from build123d import *

# Parameters (mm, degrees)
F0_W     = 40
F0_H     = 40
F1_DEPTH = 1550
F2_R     = 6.5
F3_DEPTH = 10
F4_R     = 6.5
F5_DEPTH = 10


with BuildPart() as f1:
    # F0 (on Top) → F1 (new body)
    with BuildSketch(Plane.XY):
        with BuildLine():
            Line((-20, -25), (20, -25))
            ThreePointArc((20, -25), (23.535534, -23.535534), (25, -20))
            Line((25, -20), (25, 20))
            ThreePointArc((25, 20), (23.535534, 23.535534), (20, 25))
            Line((20, 25), (-20, 25))
            ThreePointArc((-20, 25), (-23.535534, 23.535534), (-25, 20))
            Line((-25, 20), (-25, -20))
            ThreePointArc((-25, -20), (-23.535534, -23.535534), (-20, -25))
        make_face()
        Rectangle(F0_W, F0_H, mode=Mode.SUBTRACT)
    extrude(amount=F1_DEPTH)

    # F2 (on face) → F3 (join)
    with BuildSketch(Plane.XY.offset(1550)):
        with BuildLine():
            Line((20, 25), (-20, 25))
            ThreePointArc((-20, 25), (-23.535534, 23.535534), (-25, 20))
            Line((-25, 20), (-25, -20))
            ThreePointArc((-25, -20), (-23.535534, -23.535534), (-20, -25))
            Line((-20, -25), (20, -25))
            ThreePointArc((20, -25), (23.535534, -23.535534), (25, -20))
            Line((25, -20), (25, 20))
            ThreePointArc((25, 20), (23.535534, 23.535534), (20, 25))
        make_face()
        Circle(F2_R, mode=Mode.SUBTRACT)
    extrude(amount=F3_DEPTH)

    # F4 (on face) → F5 (join)
    with BuildSketch(Plane(origin=(0, 0, 0), x_dir=(1, 0, 0), z_dir=(0, 0, -1))):
        with BuildLine():
            ThreePointArc((-20, 25), (-23.535534, 23.535534), (-25, 20))
            Line((-25, 20), (-25, -20))
            ThreePointArc((-25, -20), (-23.535534, -23.535534), (-20, -25))
            Line((-20, -25), (75, -25))
            Line((75, -25), (75, 25))
            Line((75, 25), (-20, 25))
        make_face()
        with Locations((50, 0)):
            Circle(F4_R, mode=Mode.SUBTRACT)
    extrude(amount=F5_DEPTH)


solid = f1.part
Input: part model. Units: mm. Frame: model coordinates. A direction names the side the tool comes from. Coordinates: 2 decimals unless noted, no trailing zeros. Order: outer loops, then holes, each group sorted by start corner. A loop starts at its lowest first (then second) coordinate and runs counter-clockwise, first axis right, second up.
1. Draft query along Y for faces 3 (the flat face through (-20, 0, 764)), 4 (the flat face through (25, 0, 769)), 5 (the flat face through (-5, 25, 786)). Return one class per face: +Y half, -Y half, draft (parallel to the pull), parting line (faces both ways), or undercut.
Checked values:
face 3: undercut
face 4: draft
face 5: +Y half
2. Access query for faces 1 (the flat face through (20, 0, 764)), 2 (the flat face through (-4, -25, 786)). Directions: +Z, -Z, +X, -X, +Y, -Y. A direction counts if a zero-diameter tool reaches every point of the face in a straight line with its end or side. Return the directions, or none.
Checked values:
face 1: none
face 2: +Z, -Z, +X, -X, -Y
3. Cut plane A-A, the plane z = 1399. Return loops of the section in (x, y), plus the area to 3 significant figures.
Checked values:
outline: (-25, -20) arc R5 ccw to (-20, -25) - (20, -25) arc R5 ccw to (25, -20) - (25, 20) arc R5 ccw to (20, 25) - (-20, 25) arc R5 ccw to (-25, 20) - close; hole (-20, -20) - (20, -20) - (20, 20) - (-20, 20) - close
area: 879 mm2
4. Ray query, line 1 along X through (y, z) = (-2.5, 588); line 2 along Y through (x, z) = (50, -3). Return the intervals inside material, ascending.
Checked values:
line 1: x = -25 to -20, 20 to 25
line 2: y = -25 to -6.5, 6.5 to 25
5. Contact query for flat-ended pins moving along their axis: P1, Ø3, axis at y = 7, z = 1231, coming from the +X side; P2, Ø5, axis at x = 23, z = 235, coming from the +Y side; P3, Ø25, axis at x = 53.5, y = 12, coming from the +Z side. Output: stop coordinate, or through.
Checked values:
P1: stops at x = 25
P2: stops at y = 24.97
P3: stops at z = 0
